```python
from build123d import *

# Parameters (mm, degrees)
SKETCH2_R           = 3.175
BOSS_EXTRUDE1_DEPTH = 9.525
SKETCH4_W           = 12.7
SKETCH4_H           = 27.0197796
SKETCH9_W           = 12.7
SKETCH9_H           = 27.0197796
SKETCH4_86_W        = 12.7
SKETCH4_86_H        = 27.0197796
SKETCH9_5_W         = 12.7
SKETCH9_5_H         = 27.0197796
SKETCH11_W          = 85.660440798
SKETCH11_H          = 27.0197796
BOSS_EXTRUDE3_DEPTH = 12.7
FILLET2_R           = 2.54
SKETCH12_W          = 101.6
SKETCH12_H          = 6.35
BOSS_EXTRUDE4_DEPTH = 127
FILLET4_R           = 2.54


with BuildPart() as part:
    # Sketch2 → Boss-Extrude1 (new body)
    with BuildSketch(Plane.XY):
        with BuildLine():
            Line((6.501621467, 69.546757065), (13.5098898, 55.530220399))
            ThreePointArc((13.5098898, 55.530220399), (40.411152545, 40.411152545), (55.530220399, 13.5098898))
            Line((55.530220399, 13.5098898), (69.546757065, 6.501621467))
            ThreePointArc((69.546757065, 6.501621467), (69.85, 0), (69.546757065, -6.501621467))
            Line((69.546757065, -6.501621467), (55.530220399, -13.5098898))
            ThreePointArc((55.530220399, -13.5098898), (40.411152545, -40.411152545), (13.5098898, -55.530220399))
            Line((13.5098898, -55.530220399), (6.501621467, -69.546757065))
            ThreePointArc((6.501621467, -69.546757065), (0, -69.85), (-6.501621467, -69.546757065))
            Line((-6.501621467, -69.546757065), (-13.5098898, -55.530220399))
            ThreePointArc((-13.5098898, -55.530220399), (-40.411152545, -40.411152545), (-55.530220399, -13.5098898))
            Line((-55.530220399, -13.5098898), (-69.546757065, -6.501621467))
            ThreePointArc((-69.546757065, -6.501621467), (-69.85, 0), (-69.546757065, 6.501621467))
            Line((-69.546757065, 6.501621467), (-55.530220399, 13.5098898))
            ThreePointArc((-55.530220399, 13.5098898), (-40.411152545, 40.411152545), (-13.5098898, 55.530220399))
            Line((-13.5098898, 55.530220399), (-6.501621467, 69.546757065))
            ThreePointArc((-6.501621467, 69.546757065), (0, 69.85), (6.501621467, 69.546757065))
        make_face()
        with Locations((-63.5, 0)):
            Circle(SKETCH2_R, mode=Mode.SUBTRACT)
        with Locations((0, 63.5)):
            Circle(SKETCH2_R, mode=Mode.SUBTRACT)
        with Locations((63.5, 0)):
            Circle(SKETCH2_R, mode=Mode.SUBTRACT)
        with Locations((0, -63.5)):
            Circle(SKETCH2_R, mode=Mode.SUBTRACT)
    extrude(amount=BOSS_EXTRUDE1_DEPTH)

    # Sketch4 → Loft5 section 0
    with BuildSketch(Plane.XY.offset(9.525)):
        with Locations((-42.830220399, 0)):
            Rectangle(SKETCH4_W, SKETCH4_H)
    # Sketch9 → Loft5 section 1
    with BuildSketch(Plane.XY.offset(55.245)):
        with Locations((-36.480220399, 0)):
            Rectangle(SKETCH9_W, SKETCH9_H)
    loft()

    # Sketch4<86> → Loft6 section 0
    with BuildSketch(Plane.XY.offset(9.525)):
        with Locations((42.830220399, 0)):
            Rectangle(SKETCH4_86_W, SKETCH4_86_H)
    # Sketch9<5> → Loft6 section 1
    with BuildSketch(Plane.XY.offset(55.245)):
        with Locations((36.480220399, 0)):
            Rectangle(SKETCH9_5_W, SKETCH9_5_H)
    loft()

    # Sketch11 → Boss-Extrude3 (add)
    with BuildSketch(Plane.XY.offset(55.245)):
        Rectangle(SKETCH11_W, SKETCH11_H)
    extrude(amount=-BOSS_EXTRUDE3_DEPTH)

    # Fillet2
    fillet2_edges = [part.edges().sort_by_distance(p)[0] for p in [
        (-31.894109288, 0, 42.545),
        (31.894109288, 0, 42.545),
        (-42.830220399, 0, 55.245),
        (-49.180220399, 0, 9.525),
        (-36.480220399, 0, 9.525),
        (36.480220399, 0, 9.525),
        (42.830220399, 0, 55.245),
        (49.180220399, 0, 9.525),
    ]]
    fillet(fillet2_edges, radius=FILLET2_R)

    # Sketch12 → Boss-Extrude4 (add)
    with BuildSketch(Plane(origin=(0, 0, 0), x_dir=(-1, 0, 0), z_dir=(0, 0, -1))):
        Rectangle(SKETCH12_W, SKETCH12_H)
    extrude(amount=BOSS_EXTRUDE4_DEPTH)

    # Fillet4
    fillet4_edges = [part.edges().sort_by_distance(p)[0] for p in [
        (-50.8, 0, 0),
        (50.8, 0, 0),
        (-50.8, 0, -127),
        (50.8, 0, -127),
    ]]
    fillet(fillet4_edges, radius=FILLET4_R)


solid = part.part
```
Geometry check sheet. Reference: the model listing, model coordinates, mm. A direction names the side the tool comes from. Give positions to 0.01 mm unless a question says otherwise; leave off trailing zeros. Order: outer loops, then holes, each group sorted by start corner. A loop starts at its lowest first (then second) coordinate and runs counter-clockwise, first axis right, second up.
1. Section check D-D, the plane x = 0. Enter the section's corners in (y, z) (3 decimals).
2. Access from +Z, -Z, +X, -X, +Y, -Y to the whole of each face (thin tool, end or side, straight path). Record for faces 4 (the face through (-34.11, -0.19, 26.58)), 5 (the face through (50.8, 0, -63)), 6 (the face through (1, -13.51, 45)), 7 (the face through (1, 3.175, -63)).
3. Release check for a two-part mould opening along Z. For faces 1 (the face through (-1, 0, 55.245)), 2 (the face through (0, 0, 42.545)), 3 (the face through (-9.957, -62.637, 4.696)) record: pulls with the +Z half, pulls with the -Z half, needs draft (parallel to the pull), parting line crosses it, or undercut.
4. Section check B-B, the plane x = -63.5. Enter the section's corners in (y, z) (3 decimals).
5. Thickness scan on L1, parallel to Y at x = 0, z = 6 (3 decimals); L2, parallel to Z at x = 6, y = 9.5 (3 decimals); L3, parallel to Z at x = -26.5, y = 39 (3 decimals). Record the ranges inside material, lowest first.
6. Section check A-A, the plane z = 3. Enter the section's corners in (x, y) (3 decimals).
7. Gauge pin test, flat ends, axial feed: pin 1 Ø8.5 at (x, y) = (0, -63.5) entering from +Z (3 decimals); pin 2 Ø8 at (y, z) = (22.5, 9) entering from +X; pin 3 Ø7.5 at (x, y) = (0, 63.5) entering from -Z; pin 4 Ø23 at (x, z) = (-20.5, 23) entering from +Y. Record the tip position at first contact, or that the pin passes through.
8. Section check C-C, the plane y = 0. Give the number of separate pieces and of enclosed holes in the cut face, and give its area (3 significant figures).
Values follow:
1. outline: (-69.85, 0) - (-66.675, 0) - (-66.675, 9.525) - (-69.85, 9.525) - close; (-60.325, 0) - (-3.175, 0) - (-3.175, -127) - (3.175, -127) - (3.175, 0) - (60.325, 0) - (60.325, 9.525) - (-60.325, 9.525) - close; (-13.51, 42.545) - (13.51, 42.545) - (13.51, 55.245) - (-13.51, 55.245) - close; (66.675, 0) - (69.85, 0) - (69.85, 9.525) - (66.675, 9.525) - close
2. face 4: +Y, -Y
2. face 5: -Z, +X, +Y, -Y
2. face 6: +Z, +X, -X, -Y
2. face 7: -Z, +X, -X, +Y
3. face 1: pulls with the +Z half
3. face 2: undercut
3. face 3: needs draft
4. outline: (-9.525, 0) - (-3.175, 0) - (-3.175, 9.525) - (-9.525, 9.525) - close; (3.175, 0) - (9.525, 0) - (9.525, 9.525) - (3.175, 9.525) - close
5. L1: y = -69.85 to -66.675, -60.325 to 60.325, 66.675 to 69.85
5. L2: z = 0 to 9.525, 42.545 to 55.245
5. L3: z = 0 to 9.525
6. outline: (-69.547, -6.502) - (-55.53, -13.51) arc R57.15 ccw to (-13.51, -55.53) - (-6.502, -69.547) arc R69.85 ccw to (6.502, -69.547) - (13.51, -55.53) arc R57.15 ccw to (55.53, -13.51) - (69.547, -6.502) arc R69.85 ccw to (69.547, 6.502) - (55.53, 13.51) arc R57.15 ccw to (13.51, 55.53) - (6.502, 69.547) arc R69.85 ccw to (-6.502, 69.547) - (-13.51, 55.53) arc R57.15 ccw to (-55.53, 13.51) - (-69.547, 6.502) arc R69.85 ccw to start; hole circle Ø6.35 at (-63.5, 0); hole circle Ø6.35 at (0, -63.5); hole circle Ø6.35 at (0, 63.5); hole circle Ø6.35 at (63.5, 0)
7. pin 1: stops at z = 9.525
7. pin 2: stops at x = 54.07
7. pin 3: stops at z = 0
7. pin 4: passes through
8. separate pieces: 3
8. enclosed holes: 1
8. area: 16,100 mm2
